Verification items for the finished model (mm, model axes). A direction names the side the tool comes from. Give positions to 0.01 mm unless a question says otherwise; leave off trailing zeros. Write each loop counter-clockwise with the first axis right and the second up, starting at its lowest first coordinate (ties: lowest second). Pieces come first, ordered by that corner, then holes. Notation, with made-up numbers: (-17.75, 10) - (30.25, 10) arc R37 ccw to (30.25, 47) - close; hole circle Ø11 at (48, 42.25). An arc over 180 degrees is marked (long way). Put each result on its own line as item: value.
from build123d import *

# Parameters (mm, degrees)
BOSS_EXTRUDE1_DEPTH = 50
FILLET1_R           = 2
CUT_EXTRUDE1_REACH  = 58.338
CHAMFER1_SIZE       = 0.5


with BuildPart() as part:
    # Sketch1 → Boss-Extrude1 (new body)
    with BuildSketch(Plane.XY):
        Polygon((4, 25), (-3, 25), (-3, 21), (0, 21), (0, 0), (4, 0), align=None)
    extrude(amount=BOSS_EXTRUDE1_DEPTH)

    # Fillet1
    fillet1_edges = [part.edges().sort_by_distance(p)[0] for p in [
        (-3, 25, 25),
        (4, 25, 25),
    ]]
    fillet(fillet1_edges, radius=FILLET1_R)

    # Sketch2 → Cut-Extrude1 (cut, up to next)
    with BuildSketch(Plane(origin=(4, 0, 0), x_dir=(0, 0, -1), z_dir=(1, 0, 0)), mode=Mode.PRIVATE) as cut_extrude1_sk1:
        with BuildLine():
            Line((-40, 3), (-40, 5))
            ThreePointArc((-40, 5), (-42, 7), (-44, 5))
            Line((-44, 5), (-44, 3))
            ThreePointArc((-44, 3), (-42, 1), (-40, 3))
        make_face()
    cut_extrude1_tool1 = extrude(cut_extrude1_sk1.sketch, amount=-CUT_EXTRUDE1_REACH, mode=Mode.PRIVATE) & part.part
    # Sketch2 → Cut-Extrude1 (cut, up to next)
    with BuildSketch(Plane(origin=(4, 0, 0), x_dir=(0, 0, -1), z_dir=(1, 0, 0)), mode=Mode.PRIVATE) as cut_extrude1_sk2:
        with BuildLine():
            ThreePointArc((-10, 5), (-8, 7), (-6, 5))
            Line((-6, 5), (-6, 3))
            ThreePointArc((-6, 3), (-8, 1), (-10, 3))
            Line((-10, 3), (-10, 5))
        make_face()
    cut_extrude1_tool2 = extrude(cut_extrude1_sk2.sketch, amount=-CUT_EXTRUDE1_REACH, mode=Mode.PRIVATE) & part.part
    add(cut_extrude1_tool1.solids().sort_by_distance((4, 4, 42))[0], mode=Mode.SUBTRACT)
    add(cut_extrude1_tool2.solids().sort_by_distance((4, 4, 8))[0], mode=Mode.SUBTRACT)

    # Chamfer1
    chamfer1_edges = [part.edges().sort_by_distance(p)[0] for p in [
        (4, 4, 44),
        (4, 4, 40),
        (4, 7, 42),
        (4, 1, 42),
        (4, 7, 8),
        (4, 1, 8),
        (4, 4, 10),
        (4, 4, 6),
    ]]
    chamfer(chamfer1_edges, length=CHAMFER1_SIZE)


solid = part.part
Q1. Section check B-B, the plane z = 35.5. Record the cut outline in (x, y), plus the area to 3 significant figures.
Answers follow:
outline: (-3, 21) - (0, 21) - (0, 0) - (4, 0) - (4, 23) arc R2 ccw to (2, 25) - (-1, 25) arc R2 ccw to (-3, 23) - close
area: 110 mm2
Q2. Set-up check for faces 4 (the face through (0, 11, 25)), 5 (the face through (2, 4, 40)), 6 (the face through (3.4, 24.43, 25.35)), 7 (the face through (1, 15, 50)), 8 (the face through (3.635, 0.865, 42.047)): record each of +Z, -Z, +X, -X, +Y, -Y from which the full face is reachable in a straight line by a thin tool's end or side.
Answers follow:
face 4: +Z, -Z, -X, -Y
face 5: +X, -X
face 6: +Z, -Z, +X, +Y
face 7: +Z, +X, -X, +Y, -Y
face 8: +X
Q3. Section check C-C, the plane y = 6.5. Give the number of separate pieces and of enclosed holes in the cut face, plus the area to 3 significant figures.
Answers follow:
separate pieces: 3
enclosed holes: 0
area: 178 mm2
Q4. Section check A-A, the plane z = 42. Record the cut outline in (x, y).
Answers follow:
outline: (-3, 21) - (0, 21) - (0, 7) - (3.5, 7) - (4, 7.5) - (4, 23) arc R2 ccw to (2, 25) - (-1, 25) arc R2 ccw to (-3, 23) - close; (0, 0) - (4, 0) - (4, 0.5) - (3.5, 1) - (0, 1) - close
Q5. Section check D-D, the plane y = 19.5. Record the cut outline in (x, z), plus the area to 3 significant figures.
Answers follow:
outline: (0, 0) - (4, 0) - (4, 50) - (0, 50) - close
area: 200 mm2
Q6. Release check for a two-part mould opening along Y. For faces 1 (the face through (3.635, 7.135, 8.047)), 2 (the face through (-2.4, 24.43, 25.35)), 3 (the face through (1, 15, 0)) record: released by +Y, released by -Y, zero draft, split by the parting line, or undercut.
Answers follow:
face 1: undercut
face 2: released by +Y
face 3: zero draft
Q7. Go/stop test with flat-tipped pins: pin 1 Ø6.5 at (y, z) = (6, 36.5) entering from -X; pin 2 Ø0.9 at (x, z) = (-1.5, 33.5) entering from -Y. Record where each tip stops, or that it passes through.
Answers follow:
pin 1: stops at x = 0
pin 2: stops at y = 21
Q8. Scan lines: line 1 along Z through (x, y) = (2.25, 6.25); line 2 along Y through (x, z) = (0.5, 42); line 3 along X through (y, z) = (13.5, 43). Record each from-to range of solid material in increasing order.
Answers follow:
line 1: z = 0 to 6.44, 9.56 to 40.44, 43.56 to 50
line 2: y = 0 to 1, 7 to 25
line 3: x = 0 to 4
